The listing builds one solid part. Answer for the finished solid, in the listing's coordinates (mm). A direction names the side the tool comes from. Coordinates: 2 decimals unless noted, no trailing zeros. Order: outer loops, then holes, each group sorted by start corner. A loop starts at its lowest first (then second) coordinate and runs counter-clockwise, first axis right, second up. Notation, with made-up numbers: (0, -9) -> (27, -9) arc R21 ccw to (27, -1) -> close; hole circle Ø1 at (63, 75). An arc over 180 degrees is marked (long way). Write item = value, one per line. Start each with the question number.
```python
from build123d import *

# Parameters (mm, degrees)
SKETCH_1_R      = 3.065
SKETCH_1_R_2    = 2
EXTRUDE_1_DEPTH = 3
EXTRUDE_START   = 1
SKETCH_2_R      = 3.95
SKETCH_2_R_2    = 2
EXTRUDE_2_DEPTH = 1
CHAMFER_1_SIZE  = 0.3
CHAMFER_1_SIZE2 = 0.519615242
CHAMFER_2_SIZE  = 0.2


with BuildPart() as part:
    # 草图1 → 凸台-拉伸1 (new body)
    with BuildSketch(Plane(origin=(0, 0, 0), x_dir=(1, 0, 0), z_dir=(0, 1, 0))):
        with Locations(Location((0, 0, 0), (0, 0, 270))):
            Circle(SKETCH_1_R)
        with Locations(Location((0, 0, 0), (0, 0, 270))):
            Circle(SKETCH_1_R_2, mode=Mode.SUBTRACT)
    extrude(amount=-EXTRUDE_1_DEPTH)

    # 草图2 → 凸台-拉伸2 (add)
    with BuildSketch(Plane(origin=(0, 0, 0), x_dir=(1, 0, 0), z_dir=(0, 1, 0)).offset(EXTRUDE_START)):
        with Locations(Location((0, 0, 0), (0, 0, 270))):
            Circle(SKETCH_2_R)
        with Locations(Location((0, 0, 0), (0, 0, 270))):
            Circle(SKETCH_2_R_2, mode=Mode.SUBTRACT)
    extrude(amount=-EXTRUDE_2_DEPTH)

    # 倒角1
    chamfer_1_edges = [part.edges().sort_by_distance(p)[0] for p in [
        (0, 1, -3.95),
    ]]
    chamfer_1_side = [part.faces().sort_by_distance(p)[0] for p in [
        (0, 0.5, -3.95),
    ]]
    chamfer(chamfer_1_edges, length=CHAMFER_1_SIZE, length2=CHAMFER_1_SIZE2, reference=chamfer_1_side[0])

    # 倒角2
    chamfer_2_edges = [part.edges().sort_by_distance(p)[0] for p in [
        (0, -3, -3.065),
    ]]
    chamfer(chamfer_2_edges, length=CHAMFER_2_SIZE)


solid = part.part
```
Item 1: Each of these flat-tipped pins is pushed along its axis until it touches: pin 1 (1.5 mm diameter, centred on y = -0.5, z = 1.5, fed in from +X); pin 2 (1.5 mm diameter, centred on x = -0.5, y = -1, fed in from +Z) (3 decimals). Where does it stop, or does it pass through?
Item 2: Section A-A, the plane z = 0 is taken. Give the vertices of the cut face in (x, y) (3 decimals), then the cut area to 3 significant figures.
Item 3: Section D-D, the plane y = 0.1 is taken. Give the vertices of the cut face in (x, z), then the cut area to 3 significant figures.
Item 4: For a pull along Z with two mould halves and no side action, classify faces 3 (the flat face through (2, -3, 1)), 4 (the cylindrical face through (-2, -1, 0)), 5 (the cylindrical face through (2.67, 0.35, -2.91)) as pulls with the +Z half, pulls with the -Z half, needs draft (parallel to the pull), parting line crosses it, or undercut.
Item 5: Section B-B, the plane x = 0 is taken. Give the vertices of the cut face in (y, z) (3 decimals).
Item 6: Consider probe 1 along X at (y, z) = (0.1, 0); probe 2 along X at (y, z) = (-1.15, 0) (3 decimals); probe 3 along Y at (x, z) = (-3.25, 0.25). Determine where each line is inside the solid, lowest interval first.
Item 7: Section C-C, the plane y = -1.7 is taken. Give the vertices of the cut face in (x, z) (3 decimals), then the cut area to 3 significant figures.
Item 8: Which of the six approach directions +Z, -Z, +X, -X, +Y, -Y give full straight-line access (tool end or side, diameter ignored) to faces 1 (the cylindrical face through (2.07, -1.38, -2.26)), 2 (the flat face through (0, 1, 2.2))?
A:
q1.pin_1 = 3.84
q1.pin_2 = 3.065
q2.outline = (-3.95, 0) -> (-3.065, 0) -> (-3.065, -2.8) -> (-2.865, -3) -> (-2, -3) -> (-2, 1) -> (-3.43, 1) -> (-3.95, 0.7) -> close; (2, -3) -> (2.865, -3) -> (3.065, -2.8) -> (3.065, 0) -> (3.95, 0) -> (3.95, 0.7) -> (3.43, 1) -> (2, 1) -> close
q2.area = 10.1 mm^2
q3.outline = circle Ø7.9 at (0, 0); hole circle Ø4 at (0, 0)
q3.area = 36.5 mm^2
q4.face_3 = needs draft
q4.face_4 = undercut
q4.face_5 = parting line crosses it
q5.outline = (-3, -2.865) -> (-2.8, -3.065) -> (0, -3.065) -> (0, -3.95) -> (0.7, -3.95) -> (1, -3.43) -> (1, -2) -> (-3, -2) -> close; (-3, 2) -> (1, 2) -> (1, 3.43) -> (0.7, 3.95) -> (0, 3.95) -> (0, 3.065) -> (-2.8, 3.065) -> (-3, 2.865) -> close
q6.probe_1 = -3.95 to -2, 2 to 3.95
q6.probe_2 = -3.065 to -2, 2 to 3.065
q6.probe_3 = 0 to 1
q7.outline = circle Ø6.13 at (0, 0); hole circle Ø4 at (0, 0)
q7.area = 16.9 mm^2
q8.face_1 = -Y
q8.face_2 = +Z, -Z, +X, -X, +Y
